Check sheet for the modelled part. Datum: model origin and axes. Units: mm. Round coordinates to 2 decimals unless told otherwise and drop trailing zeros. Loops run counter-clockwise (first coordinate to the right, second up) from the corner with the lowest first, then second, coordinate; pieces in that order, holes last. Notation, with made-up numbers: (56, 12) - (112, 12) arc R20 cw to (112, 23) - close; hole circle Ø5 at (7, 30). An arc over 180 degrees is marked (long way). Return JSON: item names as keys, results as strings.
from build123d import *

# Parameters (mm, degrees)
SKETCH1_W                 = 71.12
SKETCH1_H                 = 101.6
BOSS_EXTRUDE1_DEPTH       = 1.27
FILLET1_R                 = 2.794
F_4_40_TAPPED_HOLE1_D     = 2.2606
F_4_40_TAPPED_HOLE1_DEPTH = 2.286
F_4_40_TAPPED_HOLE1_TIP   = 0.679152758


with BuildPart() as part:
    # Sketch1 → Boss-Extrude1 (new body)
    with BuildSketch(Plane(origin=(0, 0, 0), x_dir=(1, 0, 0), z_dir=(0, 1, 0))):
        Rectangle(SKETCH1_W, SKETCH1_H)
    extrude(amount=BOSS_EXTRUDE1_DEPTH)

    # Fillet1
    fillet1_edges = [part.edges().sort_by_distance(p)[0] for p in [
        (35.56, 0.635, 50.8),
        (-35.56, 0.635, 50.8),
        (-35.56, 0.635, -50.8),
        (35.56, 0.635, -50.8),
    ]]
    fillet(fillet1_edges, radius=FILLET1_R)

    # #4-40 Tapped Hole1
    with Locations(Plane(origin=(0, 1.27, 0), x_dir=(1, 0, 0), z_dir=(0, 1, 0))):
        with Locations((-24.892, 45.72), (24.892, 45.72), (-24.892, -45.72), (24.892, -45.72)):
            Hole(F_4_40_TAPPED_HOLE1_D / 2, depth=F_4_40_TAPPED_HOLE1_DEPTH)
            with Locations((0, 0, -(F_4_40_TAPPED_HOLE1_DEPTH + F_4_40_TAPPED_HOLE1_TIP / 2))):  # 118° drill point
                Cone(0, F_4_40_TAPPED_HOLE1_D / 2, F_4_40_TAPPED_HOLE1_TIP, mode=Mode.SUBTRACT)


solid = part.part
Q1. Depth check by flat-ended pin: P1, Ø2.5, axis at x = -24.892, z = -45.72, coming from the -Y side. Enter the tip coordinate at first touch or a pass-through.
Answer key:
{"P1": "stops at y = 0"}
Q2. Scan line: probe 1 along X at (y, z) = (0.45, 45.72). Record every from-to range of solid material in increasing order. Write a range as [from, to].
Answer key:
{"probe 1": "x = [-35.56, -26.02], [-23.76, 23.76], [26.02, 35.56]"}
Q3. Sectioned sample at A-A (z = -45.72). Enter the section's corners in (x, y), plus the area to 3 significant figures.
Answer key:
{"outline": "(-35.56, 0) - (-26.02, 0) - (-26.02, 1.27) - (-35.56, 1.27) - close; (-23.76, 0) - (23.76, 0) - (23.76, 1.27) - (-23.76, 1.27) - close; (26.02, 0) - (35.56, 0) - (35.56, 1.27) - (26.02, 1.27) - close", "area": "84.6 mm²"}
Q4. Draft check along X on faces 1 (the face through (-34.763, 0.644, -49.96)), 2 (the face through (34.763, 0.644, -49.96)), 3 (the face through (-24.647, 0.626, 46.823)). Enter one of: released by +X, released by -X, zero draft, split by the parting line, or undercut.
Answer key:
{"face 1": "released by -X", "face 2": "released by +X", "face 3": "undercut"}
